Input: part model. Units: mm. Frame: model coordinates. Face numbers are marked on the shaded views. Coordinates: 2 decimals unless noted, no trailing zeros. Write each loop counter-clockwise with the first axis right and the second up, starting at its lowest first coordinate (ties: lowest second). Pieces come first, ordered by that corner, then holes. Notation, with made-up numbers: (28.5, 58.25) -> (75.5, 58.25) arc R35 ccw to (75.5, 90.25) -> close; hole circle Ø11 at (41, -18.5). An arc over 180 degrees is marked (long way). One line per question, with ' | ' between items. Start each with the question number.
```python
from build123d import *

# Parameters (mm, degrees)
SKETCH1_R           = 35
SKETCH1_R_2         = 6
BOSS_EXTRUDE1_DEPTH = 7.5
FILLET1_R           = 3


with BuildPart() as part:
    # Sketch1 → Boss-Extrude1 (new, symmetric)
    with BuildSketch(Plane.XY):
        with BuildLine():
            Line((-42.5, 0), (-11.544687954, 145.422934685))
            ThreePointArc((-11.544687954, 145.422934685), (0, 170), (11.544687954, 145.422934685))
            Line((11.544687954, 145.422934685), (42.5, 0))
            ThreePointArc((42.5, 0), (0, -42.5), (-42.5, 0))
        make_face()
        Circle(SKETCH1_R, mode=Mode.SUBTRACT)
        with Locations((0, 155)):
            Circle(SKETCH1_R_2, mode=Mode.SUBTRACT)
    extrude(amount=BOSS_EXTRUDE1_DEPTH, both=True)

    # Fillet1
    fillet1_edges = [part.edges().sort_by_distance(p)[0] for p in [
        (42.5, 0, 0),
        (-42.5, 0, 0),
        (27.022343977, 72.711467343, 7.5),
        (0, 170, 7.5),
        (-27.022343977, 72.711467343, 7.5),
        (0, -42.5, 7.5),
        (0, -42.5, -7.5),
        (-27.022343977, 72.711467343, -7.5),
        (0, 170, -7.5),
        (27.022343977, 72.711467343, -7.5),
    ]]
    fillet(fillet1_edges, radius=FILLET1_R)


solid = part.part
```
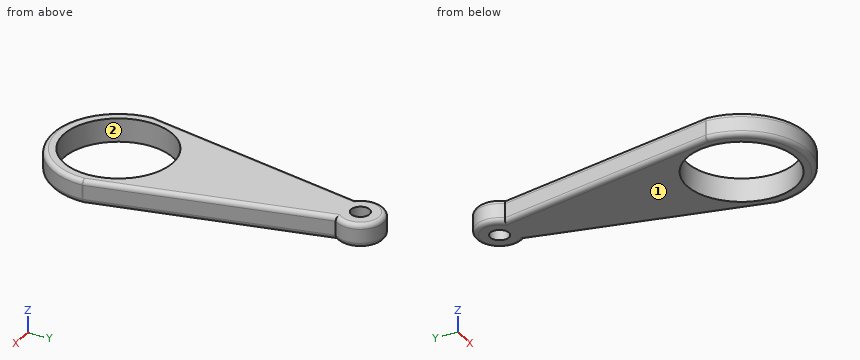
1) Ray query, line 1 (Y direction, x = 0, z = -2.5); line 2 (X direction, y = 15, z = 0.5); line 3 (Y direction, x = 9, z = -2.25). Return the intervals inside material, ascending.
2) First-contact query: P1, Ø5, axis at x = 15.5, y = 125.5, coming from the -Z side; P2, Ø8, axis at y = 42.5, z = -3, coming from the -X side; P3, Ø3, axis at y = -4, z = -2.5, coming from the +X side; P4, Ø7, axis at x = 0, y = 155, coming from the -Z side. Flat tips, straight axial feed; report the tip coordinate or a pass-through.
3) Pull-direction query (X, two-part tool) for the marked faces 1 and 2; classes: released by +X, released by -X, zero draft, split by the parting line, or undercut.
4) Section B-B, the plane z = -1. Return loops of the section in (x, y), then the cut area to 3 significant figures.
5) Section A-A, the plane x = 0. Return loops of the section in (y, z).
Answer block:
1) line 1: y = -42.5 to -35, 35 to 149, 161 to 170 | line 2: x = -39.31 to -31.62, 31.62 to 39.31 | line 3: y = -41.54 to -33.82, 33.82 to 167
2) P1: stops at z = -7.49 | P2: stops at x = -34.3 | P3: stops at x = 42.43 | P4: passes through
3) face 1: zero draft | face 2: undercut
4) outline: (-42.5, -0.33) arc R42.5 ccw to (42.5, -0.33) arc R3 ccw to (42.43, 0.31) -> (11.54, 145.42) arc R15 ccw (long way) to (-11.54, 145.42) -> (-42.43, 0.31) arc R3 ccw to start; hole circle Ø70 at (0, 0); hole circle Ø12 at (0, 155) | area: 7,350 mm2
5) outline: (-42.5, -4.5) arc R3 ccw to (-39.5, -7.5) -> (-35, -7.5) -> (-35, 7.5) -> (-39.5, 7.5) arc R3 ccw to (-42.5, 4.5) -> close; (35, -7.5) -> (149, -7.5) -> (149, 7.5) -> (35, 7.5) -> close; (161, -7.5) -> (167, -7.5) arc R3 ccw to (170, -4.5) -> (170, 4.5) arc R3 ccw to (167, 7.5) -> (161, 7.5) -> close
